Read the model definition and answer for the solid it produces. Units are mm, in the model's axes. A direction names the side the tool comes from. Give positions to 0.01 mm unless a question says otherwise; leave off trailing zeros. Order: outer loops, then holes, each group sorted by start corner. A loop starts at its lowest first (then second) coordinate and runs counter-clockwise, first axis right, second up. Notation, with made-up numbers: M 46.5,5.5 L 80.5,5.5 A22 ccw 80.5,12.5 Z; hole C 63,-37.5 d1. An arc over 180 degrees is marked long. One line per item, written item: value.
from build123d import *

# Parameters (mm, degrees)
SKETCH2_R           = 32
BOSS_EXTRUDE1_DEPTH = 10
SKETCH3_R           = 42
SKETCH3_R_2         = 32
EXTRUDE_THIN1_DEPTH = 20
SKETCH4_OUTSIDE_W   = 110.094
SKETCH4_OUTSIDE_H   = 110.094
CUT_EXTRUDE1_DEPTH  = 63.673758464
BOSS_EXTRUDE2_DEPTH = 15
SKETCH6_R           = 3
CUT_EXTRUDE2_DEPTH  = 66.665820638


with BuildPart() as part:
    # Sketch2 → Boss-Extrude1 (new body)
    with BuildSketch(Plane(origin=(0, 0, 0), x_dir=(1, 0, 0), z_dir=(0, 1, 0))):
        with Locations(Location((0, 0, 0), (0, 0, 270))):
            Circle(SKETCH2_R)
    extrude(amount=BOSS_EXTRUDE1_DEPTH)

    # Sketch3 → Extrude-Thin1 (add)
    with BuildSketch(Plane.XZ):
        Circle(SKETCH3_R)
        Circle(SKETCH3_R_2, mode=Mode.SUBTRACT)
    extrude(amount=-EXTRUDE_THIN1_DEPTH)

    # Sketch4 outside → Cut-Extrude1 (cut, through all)
    with BuildSketch(Plane.XZ):
        Rectangle(SKETCH4_OUTSIDE_W, SKETCH4_OUTSIDE_H)
        Polygon((36.373066959, -21), (36.373066959, 21), (0, 42), (-36.373066959, 21), (-36.373066959, -21), (0, -42), align=None, mode=Mode.SUBTRACT)
    extrude(amount=-CUT_EXTRUDE1_DEPTH, mode=Mode.SUBTRACT)

    # Sketch5 → Boss-Extrude2 (add)
    with BuildSketch(Plane.XZ):
        Polygon((36.373066959, 0), (18.186533479, 31.5), (-18.186533479, 31.5), (-36.373066959, 0), (-18.186533479, -31.5), (18.186533479, -31.5), align=None)
    extrude(amount=BOSS_EXTRUDE2_DEPTH)

    # Sketch6 → Cut-Extrude2 (cut, through all)
    with BuildSketch(Plane.XZ.offset(15)):
        with Locations(Location((0, 20, 0), (0, 0, 270))):
            Circle(SKETCH6_R)
        with Locations(Location((20, 0, 0), (0, 0, 270))):
            Circle(SKETCH6_R)
        with Locations(Location((0, -20, 0), (0, 0, 270))):
            Circle(SKETCH6_R)
        with Locations(Location((-20, 0, 0), (0, 0, 270))):
            Circle(SKETCH6_R)
    extrude(amount=-CUT_EXTRUDE2_DEPTH, mode=Mode.SUBTRACT)


solid = part.part
1) Find section A-A, the plane y = 8. Write down the section's boundary in (x, z).
Reported:
outline: M -36.37,-21 L 0,-42 L 36.37,-21 L 36.37,21 L 0,42 L -36.37,21 Z; hole C -20,0 d6; hole C 0,-20 d6; hole C 0,20 d6; hole C 20,0 d6
2) Find section C-C, the plane z = 19.5. Write down the section's boundary in (x, y).
Reported:
outline: M -36.37,0 L -25.11,0 L -25.11,-15 L -2.96,-15 L -2.96,10 L -25.37,10 L -25.37,20 L -36.37,20 Z; M 2.96,-15 L 25.11,-15 L 25.11,0 L 36.37,0 L 36.37,20 L 25.37,20 L 25.37,10 L 2.96,10 Z
3) Find section B-B, the plane x = 21.5. Write down the section's boundary in (y, z), plus the area to 3 significant figures.
Reported:
outline: M -15,-25.76 L 0,-25.76 L 0,-29.59 L 20,-29.59 L 20,-23.7 L 10,-23.7 L 10,-2.6 L -15,-2.6 Z; M -15,2.6 L 10,2.6 L 10,23.7 L 20,23.7 L 20,29.59 L 0,29.59 L 0,25.76 L -15,25.76 Z
area: 1,350 mm^2
4) Find section D-D, the plane y = 18. Write down the section's boundary in (x, z).
Reported:
outline: M -36.37,-21 L 0,-42 L 36.37,-21 L 36.37,21 L 0,42 L -36.37,21 Z; hole C 0,0 d64
5) Determine the mould class of faces 4 (the face through (-22.93, -2.68, 0.65)), 5 (the face through (-27.152, -7.395, 15.97)), 6 (the face through (-29, 0, 16)), 7 (the face through (17.93, 9.86, -31.65)) for opening direction Z: +Z half, -Z half, draft (parallel to the pull), parting line (faces both ways), or undercut.
Reported:
face 4: undercut
face 5: +Z half
face 6: draft
face 7: -Z half
6) Which of the six approach directions +Z, -Z, +X, -X, +Y, -Y give full straight-line access (tool end or side, diameter ignored) to faces 1 (the face through (0, 10, 0)), 2 (the face through (0, 0, 36)), 3 (the face through (31, 0, -18))?
Reported:
face 1: +Y
face 2: +Z, +X, -X, -Y
face 3: -Z, +X, -Y
7) Consider probe 1 along Z at (x, y) = (1.5, -4.5); probe 2 along Y at (x, z) = (23.5, -1); probe 3 along Z at (x, y) = (0, 17). Determine where each line is inside the solid, lowest interval first.
Reported:
probe 1: z = -31.5 to -22.6, -17.4 to 17.4, 22.6 to 31.5
probe 2: y = -15 to 10
probe 3: z = -42 to -32, 32 to 42
8) Each of these flat-tipped pins is pushed along its axis until it touches: pin 1 Ø5 at (x, z) = (-3, -39) entering from -Y; pin 2 Ø7.5 at (x, y) = (4, -7.5) entering from -Z; pin 3 Ø5 at (x, y) = (14, 7) entering from -Z; pin 4 Ø5 at (x, z) = (0, 20) entering from -Y. Where does it stop, or does it pass through?
Reported:
pin 1: stops at y = 0
pin 2: stops at z = -31.5
pin 3: stops at z = -35.36
pin 4: passes through
